Could you check a few things on this drawing? It's one solid part, dimensions in mm from its lowest x, y, z. A direction names the side the tool comes from. Coordinates: 2 decimals unless noted, no trailing zeros. Write each loop counter-clockwise with the first axis right and the second up, starting at its lowest first coordinate (ties: lowest second). Pieces come first, ordered by that corner, then holes.
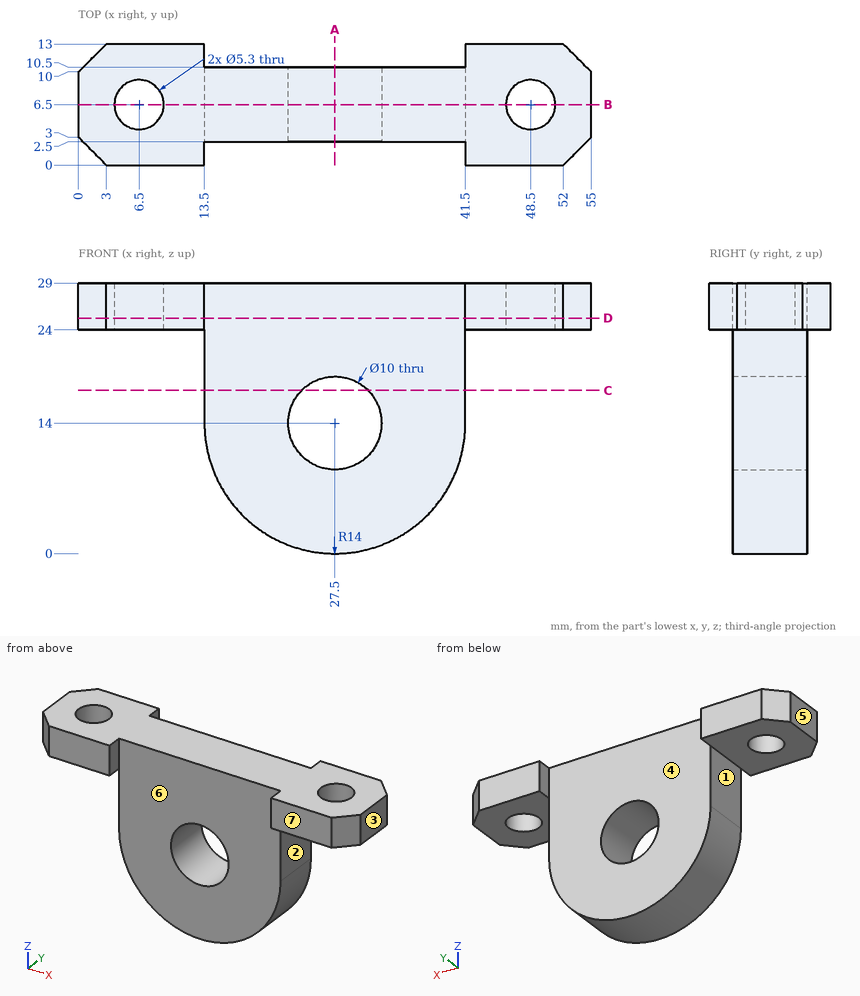
1) Imagine slicing it at A-A on x = 27.5. Please give me the cut outline in (y, z), then the cut area to 3 significant figures.
Values follow:
outline: (2.5, 0) - (10.5, 0) - (10.5, 9) - (2.5, 9) - close; (2.5, 19) - (10.5, 19) - (10.5, 29) - (2.5, 29) - close
area: 152 mm2
2) I need wall thicknesses on probe 1 along Y at (x, z) = (6.5, 25.65); probe 2 along Z at (x, y) = (27.5, 6.25); probe 3 along Z at (x, y) = (42, 9.75). Which ranges of each line are inside material? Lowest first, please.
Values follow:
probe 1: y = 0 to 3.85, 9.15 to 13
probe 2: z = 0 to 9, 19 to 29
probe 3: z = 24 to 29
3) On a 3-axis mill with a long thin cutter (end or side, diameter ignored), from which of +Z, -Z, +X, -X, +Y, -Y can I reach the whole of each face in a straight line? I mean the marked faces 1, 2, 3 and 4. Say none if no direction works.
Values follow:
face 1: -Z, -X, +Y, -Y
face 2: -Z, +X, +Y, -Y
face 3: +Z, -Z, +X, +Y, -Y
face 4: +Z, -Z, +Y
4) Imagine slicing it at D-D on z = 25.25. Please give me the cut outline in (x, y), then the cut area to 3 significant figures.
Values follow:
outline: (0, 3) - (3, 0) - (13.5, 0) - (13.5, 2.5) - (41.5, 2.5) - (41.5, 0) - (52, 0) - (55, 3) - (55, 10) - (52, 13) - (41.5, 13) - (41.5, 10.5) - (13.5, 10.5) - (13.5, 13) - (3, 13) - (0, 10) - close; hole circle Ø5.3 at (6.5, 6.5); hole circle Ø5.3 at (48.5, 6.5)
area: 513 mm2
5) Imagine slicing it at B-B on y = 6.5. Please give me the cut outline in (x, z), then the cut area to 3 significant figures.
Values follow:
outline: (0, 24) - (3.85, 24) - (3.85, 29) - (0, 29) - close; (9.15, 24) - (13.5, 24) - (13.5, 14) arc R14 ccw to (41.5, 14) - (41.5, 24) - (45.85, 24) - (45.85, 29) - (9.15, 29) - close; (51.15, 24) - (55, 24) - (55, 29) - (51.15, 29) - close; hole circle Ø10 at (27.5, 14)
area: 731 mm2
6) Imagine slicing it at C-C on z = 17.5. Please give me the cut outline in (x, y), then the cut area to 3 significant figures.
Values follow:
outline: (13.5, 2.5) - (23.93, 2.5) - (23.93, 10.5) - (13.5, 10.5) - close; (31.07, 2.5) - (41.5, 2.5) - (41.5, 10.5) - (31.07, 10.5) - close
area: 167 mm2
7) We'd pull the mould along X, two halves only. Please class the marked faces 5, 6 and 7: pulls with the +X half, pulls with the -X half, needs draft (parallel to the pull), parting line crosses it, or undercut.
Values follow:
face 5: pulls with the -X half
face 6: undercut
face 7: needs draft
8) Will these pins go through, and if not, where does the flat tip stop? pin 1 (8 mm diameter, centred on x = 26, z = 11.5, fed in from +Y); pin 2 (1.2 mm diameter, centred on y = 11.5, z = 25.5, fed in from +X); pin 3 (6.5 mm diameter, centred on y = 8.5, z = 19, fed in from -X).
Values follow:
pin 1: stops at y = 10.5
pin 2: stops at x = 54.1
pin 3: stops at x = 13.5
